For this review, take the finished solid that the model builds, in its own axes (mm). Face numbers are marked on the shaded views. Give positions to 0.01 mm unless a question says otherwise; leave off trailing zeros. Order: outer loops, then holes, each group sorted by start corner. A loop starts at its lowest first (then second) coordinate and runs counter-clockwise, first axis right, second up. Notation, with made-up numbers: M -18,45.25 L 40,45.25 A23 ccw 40,66.25 Z; hole C -27.5,76 d11. An arc over 180 degrees is marked long. Use CSV: the item, a comma, the result in double quotes. Start each with the question number.
(1) Clearance check with flat-ended pins moving along their axes: P1, Ø1, axis at y = 5.5, z = 7, coming from the -X side; P2, Ø12, axis at y = -3.5, z = 8.5, coming from the -X side; P3, Ø4, axis at y = -2.5, z = 0, coming from the -X side. State where each tip first meets the part, or that it passes through.
(2) Consider section C-C (x = 8). Write out the cut boundary in (y, z).
(3) Consider section A-A (y = 0). Write out the cut boundary in (x, z), and give its area (3 significant figures).
(4) Draft analysis for pull direction Y (two halves, no side actions). For the marked faces 1, 2 and 3, state which applies: pulls with the +Y half, pulls with the -Y half, needs draft (parallel to the pull), parting line crosses it, or undercut.
(5) Consider section B-B (z = 0). Write out the cut boundary in (x, y), and give its area (3 significant figures).
(6) Wall thickness on L1, parallel to Y at x = 8.65, z = 0; L2, parallel to Z at x = 7.25, y = 6; L3, parallel to Z at x = 8.85, y = 0: over which ranges is each line inside the solid? List them lowest first. Write a range as from..to.
(7) Consider section D-D (x = 3). Write out the cut boundary in (y, z), and give its area (3 significant figures).
```python
from build123d import *

# Parameters (mm, degrees)
F2_R      = 40
F3_DEPTH  = 17.5
F4_DEPTH  = 33
F4_FACE_R = 40
F5_DEPTH  = 80


with BuildPart() as f1:
    # F0 (on Front) → F1 (revolve)
    with BuildSketch(Plane.XZ):
        with BuildLine():
            Line((6.337865, 18), (-29.596411, 18))
            Line((-29.596411, 18), (-29.596411, 3.5))
            Line((-29.596411, 3.5), (-15.774649, 3.5))
            Line((-15.774649, 3.5), (9.337865, 3.5))
            Line((9.337865, 3.5), (9.337865, 12))
            Line((9.337865, 12), (7.337865, 12))
            ThreePointArc((7.337865, 12), (6.11312, 12.418861), (5.401373, 13.5))
            ThreePointArc((5.401373, 13.5), (6.11312, 14.581139), (7.337865, 15))
            Line((7.337865, 15), (9.337865, 15))
            ThreePointArc((9.337865, 15), (8.459185, 17.12132), (6.337865, 18))
        make_face()
        with BuildLine():
            ThreePointArc((5.337865, 14), (5.353806, 13.747991), (5.401373, 13.5))
            ThreePointArc((5.401373, 13.5), (5.353806, 13.252009), (5.337865, 13))
            Line((5.337865, 13), (5.337865, 14))
        make_face(mode=Mode.SUBTRACT)
        with BuildLine():
            ThreePointArc((5.337865, 13), (5.353806, 13.252009), (5.401373, 13.5))
            ThreePointArc((5.401373, 13.5), (5.353806, 13.747991), (5.337865, 14))
            Line((5.337865, 14), (5.337865, 13))
        make_face()
    revolve(axis=Axis((-3.107623, 0, 0), (1, 0, 0)))

    # F2 (on Front) → F3 (cut, symmetric)
    with BuildSketch(Plane.XZ):
        with Locations((-35.662135, 0)):
            Circle(F2_R)
    extrude(amount=F3_DEPTH, both=True, mode=Mode.SUBTRACT)

    # F2 (on Front) → F4 (join, symmetric)
    with BuildSketch(Plane.XZ):
        with Locations((-35.662135, 0)):
            Circle(F2_R)
    extrude(amount=F4_DEPTH, both=True)

    # F4_face (on face) → F5 (cut)
    with BuildSketch(Plane(origin=(-35.662135, -33, 0), x_dir=(1, 0, 0), z_dir=(0, -1, 0))):
        Circle(F4_FACE_R)
    extrude(amount=-F5_DEPTH, mode=Mode.SUBTRACT)


solid = f1.part
```
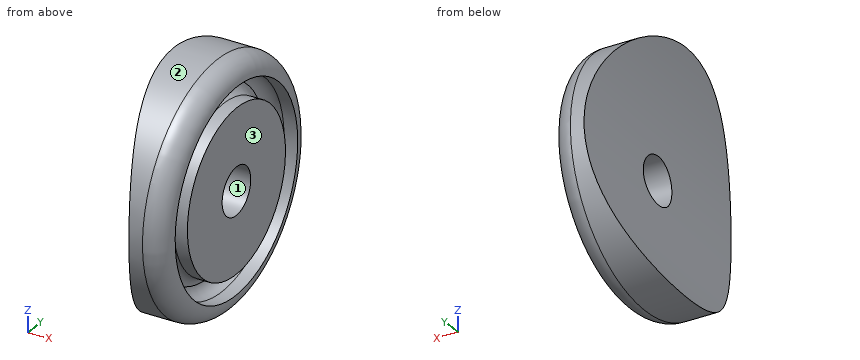
Check result:
1,P1,"stops at x = 3.63"
1,P2,"stops at x = 1.62"
1,P3,"stops at x = 4.29"
2,outline,"C 0,0 d34.99; C 0,0 d24; hole C 0,0 d30; hole C 0,0 d7"
3,outline,"M 0.06,-18 L 6.34,-18 A3 ccw 9.34,-15 L 7.34,-15 A2 cw 5.4,-13.5 A2 cw 7.34,-12 L 9.34,-12 L 9.34,-3.5 L 4.18,-3.5 A40 cw Z; M 0.06,18 A40 cw 4.18,3.5 L 9.34,3.5 L 9.34,12 L 7.34,12 A2 cw 5.4,13.5 A2 cw 7.34,15 L 9.34,15 A3 ccw 6.34,18 Z"
3,area,"170 mm^2"
4,face 1,"undercut"
4,face 2,"parting line crosses it"
4,face 3,"needs draft"
5,outline,"M 4.34,-18 L 6.34,-18 A3 ccw 9.34,-15 L 7.34,-15 A2 cw 5.4,-13.5 A2 cw 7.34,-12 L 9.34,-12 L 9.34,-3.5 L 4.34,-3.5 Z; M 4.34,3.5 L 9.34,3.5 L 9.34,12 L 7.34,12 A2 cw 5.4,13.5 A2 cw 7.34,15 L 9.34,15 A3 ccw 6.34,18 L 4.34,18 Z"
5,area,"121 mm^2"
6,L1,"y = -16.91..-15, -12..-3.5, 3.5..12, 15..16.91"
6,L2,"z = -16.82..-13.75, -10.39..10.39, 13.75..16.82"
6,L3,"z = -16.64..-15, -12..-3.5, 3.5..12, 15..16.64"
7,outline,"M -14.79,-10.26 A18 ccw 14.79,-10.26 Z; M -14.79,10.26 L 14.79,10.26 A18 ccw Z"
7,area,"321 mm^2"
